Design review of the part built by this model. Coordinates are the model's own, in mm. Face numbers are marked on the shaded views. Coordinates: 2 decimals unless noted, no trailing zeros. Write each loop counter-clockwise with the first axis right and the second up, starting at its lowest first coordinate (ties: lowest second). Pieces come first, ordered by that corner, then holes.
Q1. Take a section at C-C (z = 3.75). Give the boundary of the cut face in (x, y), and give its area (3 significant figures).
Q2. Mouldability with a two-part tool opening along Z and no side actions: class the marked faces 1 and 2 as pulls with the +Z half, pulls with the -Z half, needs draft (parallel to the pull), parting line crosses it, or undercut.
Q3. Insertion check: pin 1 (0.6 mm diameter, centred on x = 122.5, z = 1, fed in from +Y); pin 2 (12.5 mm diameter, centred on x = 163.5, y = 17, fed in from +Z); pin 3 (1.2 mm diameter, centred on x = 190, z = 2, fed in from -Y); pin 4 (1 mm diameter, centred on x = 186, z = 2, fed in from -Y). Each pin has a flat end and moves straight along its axis. Give the tip position at first contact, or say it passes through.
Q4. For probe 1 along Y at (x, z) = (201.5, -0.25); probe 2 along Z at (x, y) = (159.5, 21); probe 3 along Y at (x, z) = (190.5, 1.75), list the stretches that pass through material, from the lowest coordinate up.
Q5. Take a section at B-B (y = 10.5). Give the boundary of the cut face in (x, z).
Q6. Take a section at A-A (x = 190). Give the boundary of the cut face in (y, z), and give its area (3 significant figures).
```python
from build123d import *

# Parameters (mm, degrees)
BOX003_W        = 94
BOX003_H        = 2
BOX003_DEPTH    = 3
BOX002_W        = 100
BOX002_H        = 42
BOX002_DEPTH    = 6
SKETCH013_W     = 2
SKETCH013_H     = 10
POCKET006_DEPTH = 2
SKETCH015_W     = 2
SKETCH015_H     = 6
PAD007_DEPTH    = 2
SKETCH021_W     = 4
SKETCH021_H     = 4
PAD011_DEPTH    = 6


with BuildPart() as cube003:
    # Box003 → Box003 (new body)
    with BuildSketch(Plane(origin=(123, 4, -3), x_dir=(1, 0, 0), z_dir=(0, 0, 1))):
        with Locations((47, 1)):
            Rectangle(BOX003_W, BOX003_H)
    extrude(amount=BOX003_DEPTH)


with BuildPart() as roof_body:
    # Box002 → Box002 (new body)
    with BuildSketch(Plane(origin=(120, 0, -6), x_dir=(1, 0, 0), z_dir=(0, 0, 1))):
        with Locations((50, 21)):
            Rectangle(BOX002_W, BOX002_H)
    extrude(amount=BOX002_DEPTH)

    # Cut001: cut Cube003
    add(cube003.part, mode=Mode.SUBTRACT)

    # Sketch013 (on Face3 of BaseFeature) → Pocket006 (cut)
    with BuildSketch(Plane.XY):
        with Locations((217, 25)):
            Rectangle(SKETCH013_W, SKETCH013_H)
    extrude(amount=-POCKET006_DEPTH, mode=Mode.SUBTRACT)

    # Sketch015 (on Face3 of Pocket006) → Pad007 (join)
    with BuildSketch(Plane.XY):
        with Locations((123, 27)):
            Rectangle(SKETCH015_W, SKETCH015_H)
    extrude(amount=PAD007_DEPTH)

    # Sketch021 (on Face3 of Pad007) → Pad011 (join)
    with BuildSketch(Plane.XY):
        with Locations((190, 27)):
            Rectangle(SKETCH021_W, SKETCH021_H)
    extrude(amount=PAD011_DEPTH)


solid = roof_body.part
```
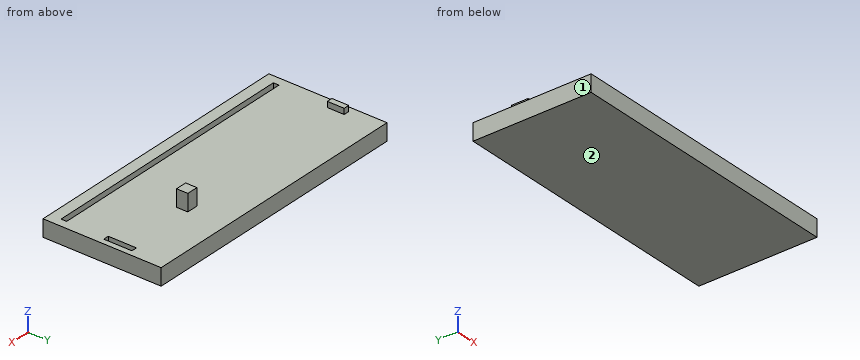
Response:
1. outline: (188, 25) - (192, 25) - (192, 29) - (188, 29) - close
1. area: 16.0 mm2
2. face 1: needs draft
2. face 2: pulls with the -Z half
3. pin 1: stops at y = 30
3. pin 2: stops at z = 0
3. pin 3: stops at y = 25
3. pin 4: passes through
4. probe 1: y = 0 to 4, 6 to 42
4. probe 2: z = -6 to 0
4. probe 3: y = 25 to 29
5. outline: (120, -6) - (220, -6) - (220, 0) - (120, 0) - close
6. outline: (0, -6) - (42, -6) - (42, 0) - (29, 0) - (29, 6) - (25, 6) - (25, 0) - (6, 0) - (6, -3) - (4, -3) - (4, 0) - (0, 0) - close
6. area: 270 mm2
